Verification items for this drawing (mm, ordinates from the low corner). Round coordinates to 2 decimals unless told otherwise and drop trailing zeros. Loops run counter-clockwise (first coordinate to the right, second up) from the corner with the lowest first, then second, coordinate; pieces in that order, holes last. Notation, with made-up numbers: M 82.5,79.5 L 101.5,79.5 A11 cw 101.5,93.5 Z; hole C 2.25,12 d4. An arc over 180 degrees is marked long. Answer as CSV lines item,"result".
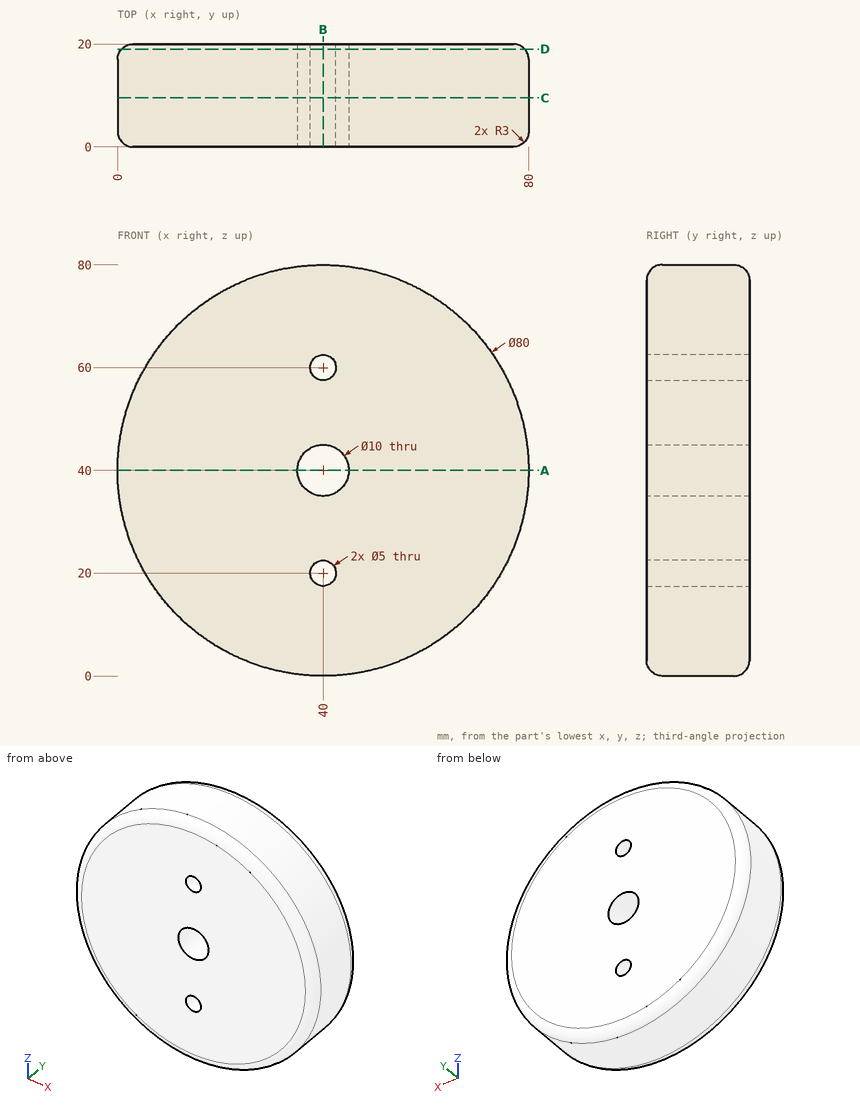
1) Go/stop test with flat-tipped pins: pin 1 (9 mm diameter, centred on x = 40, z = 40, fed in from -Y); pin 2 (10 mm diameter, centred on y = 9, z = 69.5, fed in from +X); pin 3 (3 mm diameter, centred on y = 15.5, z = 45.5, fed in from -X); pin 4 (1 mm diameter, centred on y = 4.5, z = 33, fed in from +X). Record where each tip stops, or that it passes through.
Here are the results:
pin 1,"passes through"
pin 2,"stops at x = 71.62"
pin 3,"stops at x = 0.2"
pin 4,"stops at x = 79.47"
2) Section check B-B (x = 40). Record the cut outline in (y, z).
Here are the results:
outline,"M 0,3 A3 ccw 3,0 L 17,0 A3 ccw 20,3 L 20,17.5 L 0,17.5 Z; M 0,22.5 L 20,22.5 L 20,35 L 0,35 Z; M 0,45 L 20,45 L 20,57.5 L 0,57.5 Z; M 0,62.5 L 20,62.5 L 20,77 A3 ccw 17,80 L 3,80 A3 ccw 0,77 Z"
3) Section check A-A (z = 40). Record the cut outline in (x, y).
Here are the results:
outline,"M 0,3 A3 ccw 3,0 L 35,0 L 35,20 L 3,20 A3 ccw 0,17 Z; M 45,0 L 77,0 A3 ccw 80,3 L 80,17 A3 ccw 77,20 L 45,20 Z"
4) Section check D-D (y = 19). Record the cut outline in (x, z), plus the area to 3 significant figures.
Here are the results:
outline,"C 40,40 d78.47; hole C 40,40 d10; hole C 40,20 d5; hole C 40,60 d5"
area,"4,720 mm^2"
5) Section check C-C (y = 9.5). Record the cut outline in (x, z).
Here are the results:
outline,"C 40,40 d80; hole C 40,40 d10; hole C 40,20 d5; hole C 40,60 d5"
6) Material ranges on probe 1 along Z at (x, y) = (44.5, 15.75); probe 2 along Y at (x, z) = (57.5, 7); probe 3 along X at (y, z) = (15.5, 19), recorded low to high.
Here are the results:
probe 1,"z = 0.25 to 37.82, 42.18 to 79.75"
probe 2,"y = 0.02 to 19.98"
probe 3,"x = 5.96 to 37.71, 42.29 to 74.04"
